Geometry: final body of the model. Coordinates: model frame, mm. A direction names the side the tool comes from. Coordinates: 2 decimals unless noted, no trailing zeros. Loops run counter-clockwise (first coordinate to the right, second up) from the corner with the lowest first, then second, coordinate; pieces in that order, holes last. Notation, with made-up numbers: (-34.5, -31) -> (13.5, -31) arc R11 cw to (13.5, -21) -> close; hole circle Ø1 at (-32.5, 25.25). An arc over 180 degrees is marked (long way). One line per item, written item: value. Start each with the question number.
Autodesk Inventor part; units mm, degrees
ref_plane "YZ Plane" through (0, 0, 0) normal (1, 0, 0) x (0, 1, 0)
ref_plane "XZ Plane" through (0, 0, 0) normal (0, 1, 0) x (-1, 0, 0)
ref_plane "XY Plane" through (0, 0, 0) normal (0, 0, 1) x (1, 0, 0)
sketch "Skizze1" plane through (0, 0, 0) normal (0, 0, 1) x (1, 0, 0)
  line L0 (-35.3553, 0) -> (0, 35.3553)
  line L1 (0, 35.3553) -> (35.3553, 0)
  line L2 (35.3553, 0) -> (0, -35.3553)
  line L3 (0, -35.3553) -> (-35.3553, 0)
  line L4 (-35.3553, 0) -> (35.3553, 0) construction
  line L5 (0, 35.3553) -> (0, -35.3553) construction
  point P0 (0, 0)
  point P1 (0, 0)
  dimension "d0" = 50
  dimension "d1" = 50
extrude "Extrusion1" add sketch "Skizze1" along normal mid plane 50
sketch "Skizze2" plane through (0, 0, 0) normal (0, 0, 1) x (1, 0, 0)
  line L0 (-200, 10) -> (200, 10)
  line L1 (200, 10) -> (200, -10)
  line L2 (200, -10) -> (-200, -10)
  line L3 (-200, -10) -> (-200, 10)
  line L4 (-200, 10) -> (200, -10) construction
  line L5 (200, 10) -> (-200, -10) construction
  line L6 (-10, -200) -> (-10, 200)
  line L7 (-10, 200) -> (10, 200)
  line L8 (10, 200) -> (10, -200)
  line L9 (10, -200) -> (-10, -200)
  point P0 (0, 0)
  point P1 (0, 200)
  point P2 (-10, 0)
  point P3 (0, -200)
  point P4 (-10, -10)
  point P5 (10, -10)
  point P6 (10, 10)
  point P7 (-10, 10)
  dimension "d4" = 400
  dimension "d5" = 20
  dimension "d6" = 400
  dimension "d7" = 20
extrude "Extrusion2" add sketch "Skizze2" along normal mid plane 20
sketch "Skizze3" plane through (0, 0, 0) normal (0, 0, 1) x (1, 0, 0)
  line L0 (-200, -10) -> (-200, 10)
  circle A0 centre (-200, 0) radius 20
  circle A1 centre (0, -200) radius 20
  circle A2 centre (200, 0) radius 20
  circle A3 centre (0, 200) radius 20
  point P0 (0, 0)
  dimension "d10" = 40
  dimension "d13" = 360
extrude "Extrusion3" add sketch "Skizze3" along normal mid plane 30
properties part number "drohne_model" material "PC/ABS-Kunststoff"
1. Set-up query: faces 5 (the face through (200, 0, 15)), 6 (the face through (17.43, 17.925, -0.35)), 7 (the face through (103, 10, 0)), 8 (the face through (-103, -10, 0)). Return all of +Z, -Z, +X, -X, +Y, -Y with unobstructed straight access to the full face (end or side cutting, diameter ignored); none if empty.
2. Line query: L1, parallel to X at y = 33, z = -2. Output: solid intervals per line, ascending. Write a range as [from, to].
3. Section B-B on x = 200. Return the cut outline in (y, z), plus the area to 3 significant figures.
4. Section A-A on y = -63.5. Return the cut outline in (x, z), plus the area to 3 significant figures.
5. Draft query along Y for faces 1 (the face through (0, -200, -15)), 2 (the face through (105, -10, 0)), 3 (the face through (0, -103, 10)), 4 (the face through (-105, 10, 0)). Return one class per face: released by +Y, released by -Y, zero draft, split by the parting line, or undercut.
6. Pin query (flat end, axial travel): pin 1 Ø5 at (x, z) = (134.5, -9.5) entering from -Y; pin 2 Ø12 at (x, y) = (6.5, 202.5) entering from +Z; pin 3 Ø6 at (x, y) = (-2, 102.5) entering from +Z. Return the tip coordinate at first contact, or that it passes through.
Checks:
1. face 5: +Z, +X, +Y, -Y
1. face 6: none
1. face 7: +Z, -Z, +Y
1. face 8: +Z, -Z, -Y
2. L1: [-10, 10]
3. outline: (-20, -15) -> (20, -15) -> (20, 15) -> (-20, 15) -> close
3. area: 1,200 mm²
4. outline: (-10, -10) -> (10, -10) -> (10, 10) -> (-10, 10) -> close
4. area: 400 mm²
5. face 1: zero draft
5. face 2: released by -Y
5. face 3: undercut
5. face 4: released by +Y
6. pin 1: y = -10
6. pin 2: z = 15
6. pin 3: z = 10
